```python
from build123d import *

# Parameters (mm, degrees)
CYLINDER095_R      = 1.5
CYLINDER095_DEPTH  = 21
CYLINDER094_R      = 1.5
CYLINDER094_DEPTH  = 21
CYLINDER085_R      = 1.8
CYLINDER085_DEPTH  = 12
CYLINDER088_R      = 3
CYLINDER088_DEPTH  = 1
CYLINDER089_R      = 3
CYLINDER089_DEPTH  = 1
CYLINDER087_R      = 5.5
CYLINDER087_DEPTH  = 4
CYLINDER086_R      = 5.5
CYLINDER086_DEPTH  = 4
BOX406008013_W     = 15
BOX406008013_H     = 29
BOX406008013_DEPTH = 18
CHAMFER_SIZE       = 0.5
CHAMFER001_SIZE    = 0.5


with BuildPart() as cylinder095:
    # Cylinder095 → Cylinder095 (new body)
    with BuildSketch(Plane(origin=(3, -13, -4), x_dir=(1, 0, 0), z_dir=(0, -1, 0))):
        Circle(CYLINDER095_R)
    extrude(amount=CYLINDER095_DEPTH)


with BuildPart() as fusion103077013004017014:
    # Cylinder094 → Cylinder094 (new body)
    with BuildSketch(Plane(origin=(-3, -13, -14), x_dir=(1, 0, 0), z_dir=(0, -1, 0))):
        Circle(CYLINDER094_R)
    extrude(amount=CYLINDER094_DEPTH)

    # Fusion103077013004017014: union Cylinder095
    add(cylinder095.part)


with BuildPart() as cylinder081:
    # Cylinder085 → Cylinder085 (new body)
    with BuildSketch(Plane.XY.offset(-14)):
        Circle(CYLINDER085_R)
    extrude(amount=CYLINDER085_DEPTH)


with BuildPart() as cylinder082:
    # Cylinder088 → Cylinder088 (new body)
    with BuildSketch(Plane.XY.offset(-5)):
        Circle(CYLINDER088_R)
    extrude(amount=CYLINDER088_DEPTH)


with BuildPart() as fusion103077013004017009:
    # Cylinder089 → Cylinder089 (new body)
    with BuildSketch(Plane.XY.offset(-14)):
        Circle(CYLINDER089_R)
    extrude(amount=CYLINDER089_DEPTH)

    # Fusion103077013004017009: union Cylinder082
    add(cylinder082.part)


with BuildPart() as f_623_bearing003:
    # Cylinder087 → Cylinder087 (new body)
    with BuildSketch(Plane.XY.offset(-18)):
        Circle(CYLINDER087_R)
    extrude(amount=CYLINDER087_DEPTH)


with BuildPart() as f_623_bearing_holes:
    # Cylinder086 → Cylinder086 (new body)
    with BuildSketch(Plane.XY.offset(-4)):
        Circle(CYLINDER086_R)
    extrude(amount=CYLINDER086_DEPTH)

    # Fusion103077013004017008: union 623 Bearing003
    add(f_623_bearing003.part)


with BuildPart() as cut078:
    # Box406008013 → Box406008013 (new body)
    with BuildSketch(Plane(origin=(-7.5, -22, -18), x_dir=(1, 0, 0), z_dir=(0, 0, 1))):
        with Locations((7.5, 14.5)):
            Rectangle(BOX406008013_W, BOX406008013_H)
    extrude(amount=BOX406008013_DEPTH)

    # Cut070: cut 623 Bearing Holes
    add(f_623_bearing_holes.part, mode=Mode.SUBTRACT)

    # Cut071: cut Fusion103077013004017009
    add(fusion103077013004017009.part, mode=Mode.SUBTRACT)

    # Cut072: cut Cylinder081
    add(cylinder081.part, mode=Mode.SUBTRACT)

    # Chamfer
    chamfer_edges = [cut078.edges().sort_by_distance(p)[0] for p in [
        (-3, 0, -5),
    ]]
    chamfer(chamfer_edges, length=CHAMFER_SIZE)

    # Chamfer001
    chamfer001_edges = [cut078.edges().sort_by_distance(p)[0] for p in [
        (-3, 0, -13),
    ]]
    chamfer(chamfer001_edges, length=CHAMFER001_SIZE)

    # Cut078: cut Fusion103077013004017014
    add(fusion103077013004017014.part, mode=Mode.SUBTRACT)


solid = cut078.part
```
The listing builds one solid part. Answer for the finished solid, in the listing's coordinates (mm). A direction names the side the tool comes from. Coordinates: 2 decimals unless noted, no trailing zeros. Loops run counter-clockwise (first coordinate to the right, second up) from the corner with the lowest first, then second, coordinate; pieces in that order, holes last. Notation, with made-up numbers: (21, 45.25) - (68, 45.25) arc R18 ccw to (68, 72.25) - close; hole circle Ø3 at (-20.5, 3.5). An arc over 180 degrees is marked (long way). Write item = value, one per line.
1) Section D-D (x = 3.5) is taken. Determine the outline of the cut face in (y, z).
Responses:
outline = (-22, -18) - (-4.24, -18) - (-4.24, -14) - (4.24, -14) - (4.24, -18) - (7, -18) - (7, 0) - (4.24, 0) - (4.24, -4) - (-4.24, -4) - (-4.24, 0) - (-22, 0) - (-22, -2.59) - (-13, -2.59) - (-13, -5.41) - (-22, -5.41) - close
2) Each of these flat-tipped pins is pushed along its axis until it touches: P1, Ø4, axis at x = 0, y = 0, coming from the -Z side; P2, Ø5.5, axis at x = 0.5, y = 1.5, coming from the -Z side; P3, Ø5.5, axis at x = -0.5, y = 1, coming from the +Z side. Where does it stop, or does it pass through?
Responses:
P1 = -13
P2 = -14
P3 = -4
3) Determine the mould class of faces 1 (the face through (0, -22, -9)), 2 (the face through (7.5, -8, -9)), 3 (the face through (1.717, 0.541, -9.056)) for opening direction X: pulls with the +X half, pulls with the -X half, needs draft (parallel to the pull), parting line crosses it, or undercut.
Responses:
face_1 = needs draft
face_2 = pulls with the +X half
face_3 = undercut
4) Section C-C (y = 0) is taken. Determine the outline of the cut face in (x, z), plus the area to 3 significant figures.
Responses:
outline = (-7.5, -18) - (-5.5, -18) - (-5.5, -14) - (-3, -14) - (-3, -13.5) - (-2.5, -13) - (-1.8, -13) - (-1.8, -5) - (-2.5, -5) - (-3, -4.5) - (-3, -4) - (-5.5, -4) - (-5.5, 0) - (-7.5, 0) - close; (1.8, -13) - (2.5, -13) - (3, -13.5) - (3, -14) - (5.5, -14) - (5.5, -18) - (7.5, -18) - (7.5, 0) - (5.5, 0) - (5.5, -4) - (3, -4) - (3, -4.5) - (2.5, -5) - (1.8, -5) - close
area = 142 mm^2
5) Which of the six approach directions +Z, -Z, +X, -X, +Y, -Y give full straight-line access (tool end or side, diameter ignored) to faces 4 (the face through (-3, 0.1, -4.3)), 5 (the face through (-1.614, -17.437, -14.575)), 6 (the face through (2.4, -2.4, -14))?
Responses:
face_4 = +Z
face_5 = -Y
face_6 = -Z
6) Find the intervals of material crossed by line 1 along Y through (x, z) = (0, -4.1); line 2 along Y through (x, z) = (0, -14.9); line 3 along X through (y, z) = (0, -8.5), in increasing order.
Responses:
line_1 = -22 to -3, 3 to 7
line_2 = -22 to -5.5, 5.5 to 7
line_3 = -7.5 to -1.8, 1.8 to 7.5
7) Section A-A (x = 0) is taken. Determine the outline of the cut face in (y, z).
Responses:
outline = (-22, -18) - (-5.5, -18) - (-5.5, -14) - (-3, -14) - (-3, -13.5) - (-2.5, -13) - (-1.8, -13) - (-1.8, -5) - (-2.5, -5) - (-3, -4.5) - (-3, -4) - (-5.5, -4) - (-5.5, 0) - (-22, 0) - close; (1.8, -13) - (2.5, -13) - (3, -13.5) - (3, -14) - (5.5, -14) - (5.5, -18) - (7, -18) - (7, 0) - (5.5, 0) - (5.5, -4) - (3, -4) - (3, -4.5) - (2.5, -5) - (1.8, -5) - close
8) Section B-B (z = -16.25) is taken. Determine the outline of the cut face in (x, y).
Responses:
outline = (-7.5, -22) - (7.5, -22) - (7.5, 7) - (-7.5, 7) - close; hole circle Ø11 at (0, 0)
